Autodesk Inventor part; units mm, degrees
ref_plane "Work Plane1" through (0, 0, 20) normal (1, 0, 0) x (0, 0, -1)
ref_plane "YZ Plane" through (0, 0, 0) normal (1, 0, 0) x (0, 1, 0)
ref_plane "XZ Plane" through (0, 0, 0) normal (0, 1, 0) x (-1, 0, 0)
sketch "Sketch1" plane through (0, 0, 0) normal (0, 1, 0) x (-1, 0, 0)
  line L0 (-10, -20) -> (10, -20)
  line L1 (10, -20) -> (10, 20)
  line L2 (10, 20) -> (-10, 20)
  line L3 (-10, 20) -> (-10, -20)
  line L4 (-10, -20) -> (10, 20) construction
  line L5 (10, -20) -> (-10, 20) construction
  point P0 (0, 0)
  dimension "d0" = 20
  dimension "d1" = 40
extrude "Extrusion1" add sketch "Sketch1" along normal blind 2
ref_plane "Work Plane1" through (0, 0, 20) normal (1, 0, 0) x (0, 0, -1)
sketch "Sketch3" plane through (0, 0, 20) normal (1, 0, 0) x (0, 0, -1)
  line L0 (40, 0) -> (40, 2)
  line L1 (40, 0) -> (20, 0)
  line L2 (40, 0) -> (0, 0)
  line L3 (20, 0) -> (20, -3.75)
  line L4 (20, 0) -> (23.75, 0) construction
  arc A0 (23.75, 0) -> (20, 3.75) centre (20, 0) ccw
  line L5 (20, 3.75) -> (20, 0)
  line L6 (20, 0) -> (23.75, 0)
  point P0 (20, 0)
  dimension "d5" = 20
  dimension "d6" = 3.75
  dimension "d7" = 90
  dimension "d8" = 3.75
revolve "Revolution1" cut sketch "Sketch3" angle 360 about axis through (0, 3.75, 0) along (0, -1, 0)
pattern_of_one "Rectangular Pattern1"
sketch "Sketch4" plane through (0, 2, 0) normal (0, 1, 0) x (1, 0, 0)
  line L0 (-10, -20) -> (10, -20)
  line L1 (0, -20) -> (0, -15)
  line L2 (10, 20) -> (-10, 20)
  line L3 (0, 20) -> (0, 15)
  circle A0 centre (0, -15) radius 3
  circle A1 centre (0, 15) radius 3
  point P0 (0, 0)
  dimension "d16" = 5
  dimension "d17" = 5
  dimension "d18" = 6
  dimension "d19" = 6
extrude "Extrusion2" cut sketch "Sketch4" against normal through all
fillet "Fillet1" radius 1 4 edges at (10, 2, 0) (0, 2, 20) (-10, 2, 0) (0, 2, -20)
fillet "Fillet2" radius 1 4 edges at (10, 0, 0) (0, 0, 20) (-10, 0, 0) (0, 0, -20)
fillet "Fillet3" radius 1 1 edges at (0, 0, 3.75)
properties part number "TestBearingTop"
Input: part model. Units: mm. Frame: model coordinates. Coordinates: 2 decimals unless noted, no trailing zeros. Loops run counter-clockwise (first coordinate to the right, second up) from the corner with the lowest first, then second, coordinate; pieces in that order, holes last. Notation, with made-up numbers: (80, 66.5) -> (127, 66.5) arc R19 cw to (127, 92.5) -> close; hole circle Ø11 at (19.25, 87). An arc over 180 degrees is marked (long way). Write each question's results on one line, items separated by ' | '. Start each with the question number.
Q1. Ray query, line 1 (X direction, y = 1.05, z = -15); line 2 (Z direction, x = -1.25, y = 0.75); line 3 (Z direction, x = 0, y = 0.75). Return the intervals inside material, ascending. Write a range as from..to.
Q2. Section B-B, the plane y = 1.5. Return the cut outline in (x, z), plus the area to 3 significant figures.
Q3. Section C-C, the plane x = 2.5. State how many separate pieces and enclosed holes the cut face has, plus the area to 3 significant figures.
Q4. Pull-direction query (Z, two-part tool) for faces 1 (the cylindrical face through (-9.715, 0.301, 0.28)), 2 (the cylindrical face through (0.14, 1.715, 19.699)), 3 (the cylindrical face through (-0.65, 1.01, 17.93)); classes: released by +Z, released by -Z, zero draft, split by the parting line, or undercut.
Q5. Pin query (flat end, axial travel): pin 1 (5 mm diameter, centred on x = 0, z = 15, fed in from -Y). Return the tip coordinate at first contact, or that it passes through.
Found:
1) line 1: -10..-3, 3..10 | line 2: -19.97..-17.73, -12.27..-3.46, 3.46..12.27, 17.73..19.97 | line 3: -19.97..-18, -12..-3.68, 3.68..12, 18..19.97
2) outline: (-9.87, -19.87) -> (9.87, -19.87) -> (9.87, 19.87) -> (-9.87, 19.87) -> close; hole circle Ø6.87 at (0, 0); hole circle Ø6 at (0, -15); hole circle Ø6 at (0, 15) | area: 690 mm2
3) separate pieces: 4 | enclosed holes: 0 | area: 55.3 mm2
4) face 1: zero draft | face 2: released by +Z | face 3: undercut
5) pin 1: through
